```python
from build123d import *

# Parameters (mm, degrees)
SKETCH_W        = 70
SKETCH_H        = 80
PAD_DEPTH       = 2
SKETCH001_R     = 3.5
PAD001_DEPTH    = 3
SKETCH002_R     = 1.5
PAD002_DEPTH    = 5
SKETCH003_W     = 35
SKETCH003_H     = 15
PAD003_DEPTH    = 3
PAD003_FACE12_W = 35
PAD003_FACE12_H = 3
PAD004_DEPTH    = 2
PAD004_FACE18_W = 2
PAD004_FACE18_H = 35
PAD005_DEPTH    = 3
POCKET_DEPTH    = 1
FILLET_R        = 0.2
FILLET001_R     = 4
SKETCH005_R     = 2
HOLE_DEPTH      = 25
SKETCH006_W     = 8
SKETCH006_H     = 10
PAD006_DEPTH    = 3


with BuildPart() as part:
    # Sketch → Pad (new body)
    with BuildSketch(Plane.XY):
        with Locations((35, 40)):
            Rectangle(SKETCH_W, SKETCH_H)
    extrude(amount=PAD_DEPTH)

    # Sketch001 (on Face6 of Pad) → Pad001 (join)
    with BuildSketch(Plane.XY.offset(2)):
        with Locations((11, 56)):
            Circle(SKETCH001_R)
        with Locations((61, 12)):
            Circle(SKETCH001_R)
    extrude(amount=PAD001_DEPTH)

    # Sketch002 (on Face10 of Pad001) → Pad002 (join)
    with BuildSketch(Plane.XY.offset(5)):
        with Locations((11, 56)):
            Circle(SKETCH002_R)
        with Locations((61, 12)):
            Circle(SKETCH002_R)
    extrude(amount=PAD002_DEPTH)

    # Sketch003 (on Face5 of Pad002) → Pad003 (join)
    with BuildSketch(Plane.XY.offset(2)):
        with Locations((35, 69.5)):
            Rectangle(SKETCH003_W, SKETCH003_H)
    extrude(amount=PAD003_DEPTH)

    # Pad003 Face12 → Pad004 (add)
    with BuildSketch(Plane(origin=(35, 77, 3.5), x_dir=(1, 0, 0), z_dir=(0, 1, 0))):
        Rectangle(PAD003_FACE12_W, PAD003_FACE12_H)
    extrude(amount=PAD004_DEPTH)

    # Pad004 Face18 → Pad005 (add)
    with BuildSketch(Plane(origin=(35, 78, 5), x_dir=(0, 1, 0), z_dir=(0, 0, 1))):
        Rectangle(PAD004_FACE18_W, PAD004_FACE18_H)
    extrude(amount=PAD005_DEPTH)

    # Sketch004 (on Face17 of Pad005) → Pocket (cut)
    with BuildSketch(Plane.XY.offset(5)):
        with BuildLine():
            add(Edge.make_bspline(
                [(42.5, 69.5), (42.5, 76.428203), (31.25, 72.964102), (20, 69.5), (31.25, 66.035898), (42.5, 62.571797), (42.5, 69.5)],
                knots=[0, 0, 0, 2.094395, 2.094395, 4.18879, 4.18879, 6.283185, 6.283185, 6.283185], degree=2, weights=[1, 0.5, 1, 0.5, 1, 0.5, 1]))
        make_face()
    extrude(amount=-POCKET_DEPTH, mode=Mode.SUBTRACT)

    # Fillet
    fillet_edges = [part.edges().sort_by_distance(p)[0] for p in [
        (27.500079, 69.481686, 4),
    ]]
    fillet(fillet_edges, radius=FILLET_R)

    # Fillet001
    fillet001_edges = [part.edges().sort_by_distance(p)[0] for p in [
        (0, 0, 1),
        (70, 0, 1),
        (70, 80, 1),
        (0, 80, 1),
    ]]
    fillet(fillet001_edges, radius=FILLET001_R)

    # Sketch005 (on Face1 of Fillet001) → Hole (cut)
    with BuildSketch(Plane.XY.offset(2)):
        with Locations((4, 76)):
            Circle(SKETCH005_R)
        with Locations((66, 4)):
            Circle(SKETCH005_R)
    extrude(amount=-HOLE_DEPTH, mode=Mode.SUBTRACT)

    # Sketch006 (on Face1 of Hole) → Pad006 (join)
    with BuildSketch(Plane.XY.offset(2)):
        with Locations((57, 54)):
            Rectangle(SKETCH006_W, SKETCH006_H)
        with Locations((13, 13)):
            Rectangle(SKETCH006_W, SKETCH006_H)
    extrude(amount=PAD006_DEPTH)


solid = part.part
```
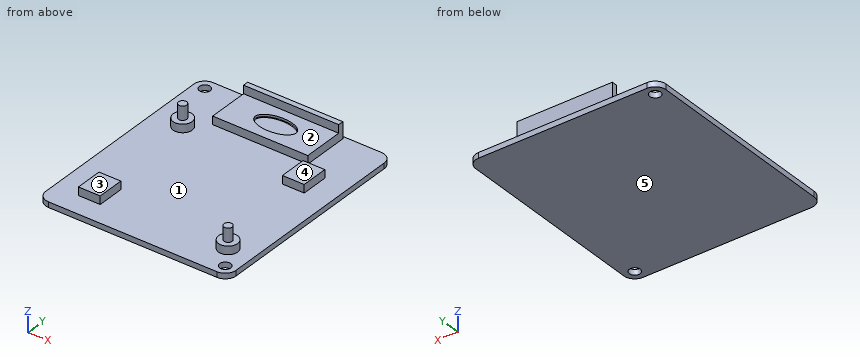
Here's how the part is built. I have some questions about the finished solid (model axes, mm). Face numbers are marked on the shaded views. A direction names the side the tool comes from. Round coordinates to 2 decimals unless told otherwise and drop trailing zeros. Write each loop counter-clockwise with the first axis right and the second up, starting at its lowest first coordinate (ties: lowest second). Pieces come first, ordered by that corner, then holes. Notation, with made-up numbers: M 26,67.5 L 61,67.5 A20 ccw 61,83.5 Z; hole C 17.5,-31.5 d7. An arc over 180 degrees is marked long. Answer as CSV lines item,"result". Start each with the question number.
1. On a 3-axis mill with a long thin cutter (end or side, diameter ignored), from which of +Z, -Z, +X, -X, +Y, -Y can I reach the whole of each face in a straight line? I mean the marked faces 3, 4 and 5. Say none if no direction works.
2. Suppose I cut it at D-D on y = 22. Write out the boundary of the cut face in (x, z).
3. I need wall thicknesses on probe 1 along Y at (x, z) = (4, 1.25); probe 2 along Y at (x, z) = (66, 1.55); probe 3 along Z at (x, y) = (33.5, 20). Which ranges of each line are inside material? Lowest first, please.
4. Suppose I cut it at C-C on x = 11. Write out the boundary of the cut face in (y, z), then the cut area to 3 significant figures.
5. I'm going to push flat-ended pins straight in: pin 1 Ø5 at (x, z) = (26.5, 8.5) entering from +Y; pin 2 Ø4 at (x, y) = (32.5, 70.5) entering from +Z; pin 3 Ø1.5 at (y, z) = (18.5, 4.5) entering from -X. Where does each tip first touch, or does it pass through?
6. Suppose I cut it at B-B on y = 56. Write out the boundary of the cut face in (x, z), then the cut area to 3 significant figures.
7. Suppose I cut it at A-A on x = 50.5. Write out the boundary of the cut face in (y, z), then the cut area to 3 significant figures.
8. Thinking about a two-plate mould opening in X: for the marked faces 1 and 2, which applies, released by +X, released by -X, zero draft, split by the parting line, or undercut?
Check result:
1,face 3,"+Z, -X, -Y"
1,face 4,"+Z, +X, +Y"
1,face 5,"-Z, +X, -X, +Y, -Y"
2,outline,"M 0,0 L 70,0 L 70,2 L 0,2 Z"
3,probe 1,"y = 0 to 74, 78 to 80"
3,probe 2,"y = 0 to 2, 6 to 80"
3,probe 3,"z = 0 to 2"
4,outline,"M 0,0 L 80,0 L 80,2 L 59.5,2 L 59.5,5 L 57.5,5 L 57.5,10 L 54.5,10 L 54.5,5 L 52.5,5 L 52.5,2 L 18,2 L 18,5 L 8,5 L 8,2 L 0,2 Z"
4,area,"226 mm2"
5,pin 1,"stops at y = 79"
5,pin 2,"stops at z = 4"
5,pin 3,"stops at x = 9"
6,outline,"M 0,0 L 70,0 L 70,2 L 61,2 L 61,5 L 53,5 L 53,2 L 14.5,2 L 14.5,5 L 12.5,5 L 12.5,10 L 9.5,10 L 9.5,5 L 7.5,5 L 7.5,2 L 0,2 Z"
6,area,"200 mm2"
7,outline,"M 0,0 L 80,0 L 80,2 L 79,2 L 79,8 L 77,8 L 77,5 L 62,5 L 62,2 L 0,2 Z"
7,area,"217 mm2"
8,face 1,"undercut"
8,face 2,"zero draft"
